Read the model definition and answer for the solid it produces. Units are mm, in the model's axes. A direction names the side the tool comes from. Give positions to 0.01 mm unless a question says otherwise; leave off trailing zeros. Write each loop counter-clockwise with the first axis right and the second up, starting at its lowest first coordinate (ties: lowest second). Pieces come first, ordered by that corner, then holes. Notation, with made-up numbers: (47, 20) - (74, 20) arc R21 cw to (74, 58) - close; hole circle Ø6 at (74.5, 81.5). An arc over 180 degrees is marked (long way). Answer as CSV lines item,"result".
```python
from build123d import *

# Parameters (mm, degrees)
F0_W     = 88.9
F0_H     = 73.025
F0_W_2   = 83.82
F0_H_2   = 67.945
F1_DEPTH = 2.54
F0_R     = 12.7
F2_DEPTH = 5.08


with BuildPart() as f1:
    # F0 (on Top) → F1 (new body)
    with BuildSketch(Plane.XY):
        with Locations((-26.052929, -38.132125)):
            Rectangle(F0_W, F0_H)
        with Locations((-25.966533, -38.132125)):
            Rectangle(F0_W_2, F0_H_2, mode=Mode.SUBTRACT)
    extrude(amount=F1_DEPTH)

    # F0 (on Top) → F2 (join)
    with BuildSketch(Plane.XY):
        with Locations((-25.966533, -38.132125)):
            Rectangle(F0_W_2, F0_H_2)
        with Locations((-28.340409, -38.598955)):
            Circle(F0_R, mode=Mode.SUBTRACT)
    extrude(amount=F2_DEPTH)


solid = f1.part
```
(1) The mould has two halves that part along X. Classify faces 1 (the flat face through (18.397, -39, 1)), 2 (the cylindrical face through (-31.094, -50.997, 2.504)), 3 (the flat face through (-30, -73, 2.54)): +X half, -X half, draft (parallel to the pull), parting line (faces both ways), or undercut.
Worked out:
face 1,"+X half"
face 2,"undercut"
face 3,"draft"
(2) For faces 4 (the flat face through (-27, -4.16, 4)), 5 (the flat face through (15.943, -39, 4)), 6 (the flat face through (-27, -72.105, 4)), determine the directions among +Z, -Z, +X, -X, +Y, -Y from which every point of the face is accessible in a straight line to the end or side of a thin tool.
Worked out:
face 4,"+Z, +X, -X, +Y"
face 5,"+Z, +X, +Y, -Y"
face 6,"+Z, +X, -X, -Y"
(3) A cutting plane is placed at B-B (x = -26.5). Write down the section's boundary in (y, z), and give its area (3 significant figures).
Worked out:
outline,"(-74.64, 0) - (-51.16, 0) - (-51.16, 5.08) - (-72.1, 5.08) - (-72.1, 2.54) - (-74.64, 2.54) - close; (-26.03, 0) - (-1.62, 0) - (-1.62, 2.54) - (-4.16, 2.54) - (-4.16, 5.08) - (-26.03, 5.08) - close"
area,"230 mm^2"
(4) A cutting plane is placed at A-A (y = -49.5). Write down the section's boundary in (x, z).
Worked out:
outline,"(-70.5, 0) - (-34.86, 0) - (-34.86, 5.08) - (-67.88, 5.08) - (-67.88, 2.54) - (-70.5, 2.54) - close; (-21.82, 0) - (18.4, 0) - (18.4, 2.54) - (15.94, 2.54) - (15.94, 5.08) - (-21.82, 5.08) - close"
(5) A cutting plane is placed at C-C (z = 3.5). Write down the section's boundary in (x, y), and give its area (3 significant figures).
Worked out:
outline,"(-67.88, -72.1) - (15.94, -72.1) - (15.94, -4.16) - (-67.88, -4.16) - close; hole circle Ø25.4 at (-28.34, -38.6)"
area,"5,190 mm^2"
(6) A cutting plane is placed at D-D (y = -60.5). Write down the section's boundary in (x, z).
Worked out:
outline,"(-70.5, 0) - (18.4, 0) - (18.4, 2.54) - (15.94, 2.54) - (15.94, 5.08) - (-67.88, 5.08) - (-67.88, 2.54) - (-70.5, 2.54) - close"
(7) Find the intervals of material crossed by L1, parallel to X at y = -39, z = 2; L2, parallel to Y at x = -14, z = 4.25; L3, parallel to X at y = -36, z = 1.65, in increasing order.
Worked out:
L1,"x = -70.5 to -41.03, -15.65 to 18.4"
L2,"y = -72.1 to -4.16"
L3,"x = -70.5 to -40.77, -15.91 to 18.4"
(8) Each of these flat-tipped pins is pushed along its axis until it touches: P1, Ø2, axis at y = -44.5, z = 4, coming from the +X side; P2, Ø1, axis at y = -43.5, z = 3.5, coming from the -X side; P3, Ø0.8, axis at x = -17, z = 3.5, coming from the -Y side. Where does it stop, or does it pass through?
Worked out:
P1,"stops at x = 15.94"
P2,"stops at x = -67.88"
P3,"stops at y = -72.1"
